from build123d import *

# Parameters (mm, degrees)
F0_W     = 120.534546
F0_H     = 116.60909
F1_DEPTH = 7.62
F2_R     = 5.08
F3_W     = 16.625449
F3_H     = 21.474546
F3_R     = 4.675549
F4_DEPTH = 25.4


with BuildPart() as f1:
    # F0 (on Top) → F1 (new body)
    with BuildSketch(Plane.XY):
        Rectangle(F0_W, F0_H)
    extrude(amount=F1_DEPTH)

    # F2
    f2_edges = [f1.edges().sort_by_distance(p)[0] for p in [
        (60.267273, -58.304545, 3.81),
        (-60.267273, -58.304545, 3.81),
        (-60.267273, 58.304545, 3.81),
        (60.267273, 58.304545, 3.81),
    ]]
    fillet(f2_edges, radius=F2_R)

    # F3 (on face) → F4 (cut)
    with BuildSketch(Plane.XY.offset(7.62)):
        with Locations((-22.629092, 0)):
            Rectangle(F3_W, F3_H)
        with Locations((22.629092, 0)):
            Rectangle(F3_W, F3_H)
        with Locations((-14.316367, 26.90091)):
            Circle(F3_R)
        with BuildLine():
            Line((40.178183, 43.560948), (17.087273, 43.560948))
            ThreePointArc((17.087273, 43.560948), (15.701819, 42.175494), (17.087273, 40.79004))
            Line((17.087273, 40.79004), (40.178183, 40.79004))
            ThreePointArc((40.178183, 40.79004), (41.563638, 42.175494), (40.178183, 43.560948))
        make_face()
        with BuildLine():
            Line((44.796359, 50.222728), (6.003633, 50.222728))
            ThreePointArc((6.003633, 50.222728), (4.618179, 48.837274), (6.003633, 47.45182))
            Line((6.003633, 47.45182), (44.796359, 47.45182))
            ThreePointArc((44.796359, 47.45182), (46.181813, 48.837274), (44.796359, 50.222728))
        make_face()
        with BuildLine():
            ThreePointArc((-6.003633, 47.45182), (-4.618179, 48.837274), (-6.003633, 50.222728))
            Line((-6.003633, 50.222728), (-44.796359, 50.222728))
            ThreePointArc((-44.796359, 50.222728), (-46.181813, 48.837274), (-44.796359, 47.45182))
            Line((-44.796359, 47.45182), (-6.003633, 47.45182))
        make_face()
        with BuildLine():
            ThreePointArc((-17.087273, 40.79004), (-15.701819, 42.175494), (-17.087273, 43.560948))
            Line((-17.087273, 43.560948), (-40.178183, 43.560948))
            ThreePointArc((-40.178183, 43.560948), (-41.563638, 42.175494), (-40.178183, 40.79004))
            Line((-40.178183, 40.79004), (-17.087273, 40.79004))
        make_face()
        with BuildLine():
            ThreePointArc((17.087273, -40.79004), (15.701819, -42.175494), (17.087273, -43.560948))
            Line((17.087273, -43.560948), (40.178183, -43.560948))
            ThreePointArc((40.178183, -43.560948), (41.563638, -42.175494), (40.178183, -40.79004))
            Line((40.178183, -40.79004), (17.087273, -40.79004))
        make_face()
        with BuildLine():
            ThreePointArc((-17.087273, -43.560948), (-15.701819, -42.175494), (-17.087273, -40.79004))
            Line((-17.087273, -40.79004), (-40.178183, -40.79004))
            ThreePointArc((-40.178183, -40.79004), (-41.563638, -42.175494), (-40.178183, -43.560948))
            Line((-40.178183, -43.560948), (-17.087273, -43.560948))
        make_face()
        with BuildLine():
            ThreePointArc((-6.003633, -50.222728), (-4.618179, -48.837274), (-6.003633, -47.45182))
            Line((-6.003633, -47.45182), (-44.796359, -47.45182))
            ThreePointArc((-44.796359, -47.45182), (-46.181813, -48.837274), (-44.796359, -50.222728))
            Line((-44.796359, -50.222728), (-6.003633, -50.222728))
        make_face()
        with BuildLine():
            ThreePointArc((6.003633, -47.45182), (4.618179, -48.837274), (6.003633, -50.222728))
            Line((6.003633, -50.222728), (44.796359, -50.222728))
            ThreePointArc((44.796359, -50.222728), (46.181813, -48.837274), (44.796359, -47.45182))
            Line((44.796359, -47.45182), (6.003633, -47.45182))
        make_face()
        with Locations((-14.316367, -26.90091)):
            Circle(F3_R)
        with Locations((14.316367, -26.90091)):
            Circle(F3_R)
        with Locations((14.316367, 26.90091)):
            Circle(F3_R)
    extrude(amount=-F4_DEPTH, mode=Mode.SUBTRACT)


solid = f1.part
Work out the finished part from the listing and answer in its coordinate system (mm). A direction names the side the tool comes from. Give positions to 0.01 mm unless a question says otherwise; leave off trailing zeros. Write each loop counter-clockwise with the first axis right and the second up, starting at its lowest first coordinate (ties: lowest second). Pieces come first, ordered by that corner, then holes. Notation, with made-up numbers: M 5,79 L 23,79 A32 ccw 23,113 Z; hole C 24.5,51.25 d11. An arc over 180 degrees is marked long. Answer as CSV lines item,"result".
Q1. A cutting plane is placed at B-B on x = 38. Write down the section's boundary in (y, z), plus the area to 3 significant figures.
A:
outline,"M -58.3,0 L -50.22,0 L -50.22,7.62 L -58.3,7.62 Z; M -47.45,0 L -43.56,0 L -43.56,7.62 L -47.45,7.62 Z; M -40.79,0 L 40.79,0 L 40.79,7.62 L -40.79,7.62 Z; M 43.56,0 L 47.45,0 L 47.45,7.62 L 43.56,7.62 Z; M 50.22,0 L 58.3,0 L 58.3,7.62 L 50.22,7.62 Z"
area,"804 mm²"
Q2. A cutting plane is placed at A-A on x = 22. Write down the section's boundary in (y, z), plus the area to 3 significant figures.
A:
outline,"M -58.3,0 L -50.22,0 L -50.22,7.62 L -58.3,7.62 Z; M -47.45,0 L -43.56,0 L -43.56,7.62 L -47.45,7.62 Z; M -40.79,0 L -10.74,0 L -10.74,7.62 L -40.79,7.62 Z; M 10.74,0 L 40.79,0 L 40.79,7.62 L 10.74,7.62 Z; M 43.56,0 L 47.45,0 L 47.45,7.62 L 43.56,7.62 Z; M 50.22,0 L 58.3,0 L 58.3,7.62 L 50.22,7.62 Z"
area,"640 mm²"
Q3. A cutting plane is placed at D-D on z = 3.5. Count the separate pieces of the cut face and the enclosed holes in it, plus the area to 3 significant figures.
A:
separate pieces,"1"
enclosed holes,"14"
area,"12,300 mm²"
Q4. Given P1, Ø8.5, axis at x = 14.32, y = 26.9, coming from the -Z side, flat-ended and moving along its own axis, determine where the tip first touches the part or whether it passes through.
A:
P1,"passes through"
Q5. Find the intervals of material crossed by probe 1 along X at (y, z) = (8.5, 4); probe 2 along Y at (x, z) = (45, 4.25); probe 3 along Y at (x, z) = (-23.5, 1.25), in increasing order. Write a range as [from, to].
A:
probe 1,"x = [-60.27, -30.94], [-14.32, 14.32], [30.94, 60.27]"
probe 2,"y = [-58.3, -50.21], [-47.47, 47.47], [50.21, 58.3]"
probe 3,"y = [-58.3, -50.22], [-47.45, -43.56], [-40.79, -10.74], [10.74, 40.79], [43.56, 47.45], [50.22, 58.3]"
Q6. A tool of negligible diameter and unlimited length cuts with its end or side. For faces 4 (the flat face through (28, -43.561, 4)), 5 (the cylindrical face through (58.819, 56.777, 3.863)), from which of +Z, -Z, +X, -X, +Y, -Y can it reach the whole face along a straight path? Write none if from no direction.
A:
face 4,"+Z, -Z"
face 5,"+Z, -Z, +X, +Y"
Q7. The mould has two halves that part along X. Classify faces 1 (the flat face through (60.267, -1, 4)), 2 (the flat face through (-1, 58.305, 4)), 3 (the cylindrical face through (-41.563, -42.145, 3.863)): +X half, -X half, draft (parallel to the pull), parting line (faces both ways), or undercut.
A:
face 1,"+X half"
face 2,"draft"
face 3,"undercut"
Q8. A cutting plane is placed at C-C on x = 8. Write down the section's boundary in (y, z).
A:
outline,"M -58.3,0 L -50.22,0 L -50.22,7.62 L -58.3,7.62 Z; M -47.45,0 L 47.45,0 L 47.45,7.62 L -47.45,7.62 Z; M 50.22,0 L 58.3,0 L 58.3,7.62 L 50.22,7.62 Z"
